Geometry: final body of the model. Coordinates: model frame, mm. Face numbers are marked on the shaded views. A direction names the side the tool comes from. Coordinates: 2 decimals unless noted, no trailing zeros. Order: outer loops, then holes, each group sorted by start corner. A loop starts at its lowest first (then second) coordinate and runs counter-clockwise, first axis right, second up. Notation, with made-up numbers: M -10,-11 L 33,-11 A18 cw 33,2 Z; hole C 61.5,62.25 d1. An arc over 180 degrees is marked long. Use CSV: the item, a comma, the result in double quotes. Start each with the question number.
1. Section query A-A on z = 21.5. State how many separate pieces and enclosed holes the cut face has, and give its area (3 significant figures).
2. Set-up query: the marked faces 4 and 5. Return all of +Z, -Z, +X, -X, +Y, -Y with unobstructed straight access to the full face (end or side cutting, diameter ignored); none if empty.
3. Material intervals for line 1 (Z direction, x = 3.3, y = 9); line 2 (Z direction, x = 1.85, y = -9); line 3 (Z direction, x = 8.5, y = -8.5), sorted ascending.
4. Section query C-C on x = 2. Return the cut outline in (y, z), and give its area (3 significant figures).
5. Pull-direction query (Z, two-part tool) for the marked faces 1, 2 and 3; classes: pulls with the +Z half, pulls with the -Z half, needs draft (parallel to the pull), parting line crosses it, or undercut.
6. First-contact query: P1, Ø15, axis at y = 0.5, z = 10, coming from the +X side; P2, Ø1, axis at x = 8.5, y = 11, coming from the +Z side; P3, Ø8, axis at x = 14, z = 6, coming from the +Y side; P4, Ø1.5, axis at x = 8.5, z = -21, coming from the +Y side. Flat tips, straight axial feed; report the tip coordinate or a pass-through.
7. Section query D-D on y = -0.5. Return the cut outline in (x, z), and give its area (3 significant figures).
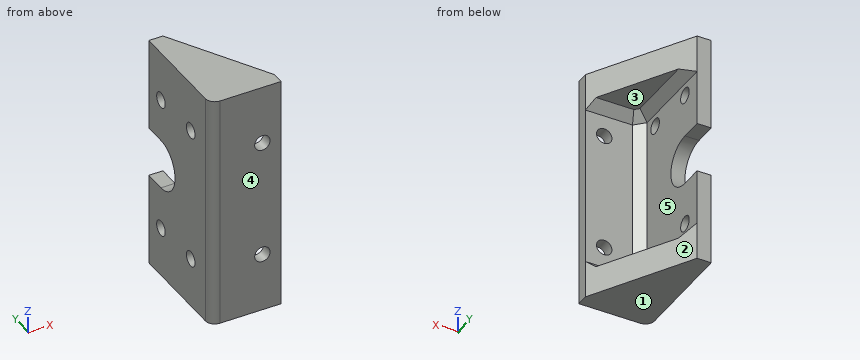
Autodesk Inventor part; units mm, degrees
ref_plane "YZ Plane" through (0, 0, 0) normal (1, 0, 0) x (0, 1, 0)
ref_plane "XZ Plane" through (0, 0, 0) normal (0, 1, 0) x (-1, 0, 0)
ref_plane "XY Plane" through (0, 0, 0) normal (0, 0, 1) x (1, 0, 0)
sketch "Sketch1" plane through (0, 0, 0) normal (1, 0, 0) x (0, 1, 0)
  line L0 (-9, -23) -> (9, -23) construction
  line L1 (9, -23) -> (9, 23) construction
  line L2 (9, 23) -> (-9, 23) construction
  line L3 (-9, 23) -> (-9, -23) construction
  line L4 (-9, -23) -> (9, 23) construction
  line L5 (9, -23) -> (-9, 23) construction
  circle A0 centre (9, 23) radius 2.6
  circle A1 centre (9, -23) radius 2.6
  circle A2 centre (-9, -23) radius 2.6
  circle A3 centre (-9, 23) radius 2.6
  circle A4 centre (9, 23) radius 7.3625 construction
  circle A5 centre (9, -23) radius 7.3625 construction
  circle A6 centre (-9, -23) radius 7.3625 construction
  circle A7 centre (-9, 23) radius 7.3625 construction
  line L6 (16.3625, 30.3625) -> (-21, 30.3625)
  line L7 (-21, 30.3625) -> (-21, -30.3625)
  line L8 (-21, -30.3625) -> (16.3625, -30.3625)
  line L9 (16.3625, -30.3625) -> (16.3625, 30.3625)
  point P0 (0, 0)
  dimension "d0" = 5.2
  dimension "d1" = 46
  dimension "d2" = 18
  dimension "d3" = 4.7625
  dimension "d7" = 12
extrude "Extrusion1" add sketch "Sketch1" along normal blind 4.7625
sketch "Sketch4" plane through (4.7625, 0, 0) normal (1, 0, 0) x (0, 0, -1)
  arc A0 (-8.5, 9) -> (8.5, 9) centre (0, 9) ccw
  circle A1 centre (-23, 9) radius 2.6
  line L0 (8.5, 9) -> (8.5, 16.3625)
  line L1 (30.3625, 16.3625) -> (-30.3625, 16.3625)
  line L2 (-8.5, 9) -> (-8.5, 16.3625)
  point P0 (0, 0)
  point P1 (27.1875, 16.3625)
  point P2 (-27.1875, 16.3625)
  dimension "d21" = 17
extrude "Extrusion5" cut sketch "Sketch4" against normal through all contours L2 L1 L0 A0
sketch "Sketch5" plane through (4.7625, 0, 0) normal (1, 0, 0) x (0, 0, -1)
  line L0 (30.3625, 16.3625) -> (8.5, 16.3625)
  line L1 (-30.3625, 16.3625) -> (-30.3625, -21)
  line L2 (-30.3625, -21) -> (30.3625, -21)
  line L3 (30.3625, -21) -> (30.3625, 16.3625)
  line L4 (-8.5, 16.3625) -> (-30.3625, 16.3625)
  line L5 (8.5, 16.3625) -> (8.5, 9)
  arc A0 (-8.5, 9) -> (8.5, 9) centre (0, 9) ccw
  line L6 (-8.5, 9) -> (-8.5, 16.3625)
  circle A1 centre (-23, -9) radius 2.6
  circle A2 centre (23, -9) radius 2.6
  circle A3 centre (23, 9) radius 2.6
  circle A4 centre (-23, 9) radius 2.6
  line L7 (30.3625, -21) -> (30.3625, 13.1875)
  line L8 (-30.3625, -21) -> (30.3625, -21)
  line L9 (30.3625, -21) -> (30.3625, -17)
  line L10 (30.3625, -17) -> (-30.3625, -17)
  line L11 (-30.3625, -17) -> (-30.3625, -21)
  point P0 (0, 0)
  point P1 (30.3625, -17.825)
  point P2 (30.3625, -17)
  point P3 (-30.3625, -17)
  dimension "d29" = 4
extrude "Extrusion6" add sketch "Sketch5" along normal blind 19.05 contours L3 L2 L1 L10
sketch "Sketch6" plane through (4.7625, -17, 30.3625) normal (0, 1, 0) x (1, 0, 0)
  circle A0 centre (12.7, 10.3625) radius 2.6
  circle A1 centre (12.7, 50.3625) radius 2.6
  line L0 (0, 9.9625) -> (0, 4.7625)
  line L1 (0, 0) -> (0, 60.725)
  line L2 (19.05, 60.725) -> (19.05, 0)
  point P0 (-4.7625, 30.3625)
  point P1 (19.05, 30.3625)
  point P2 (19.05, 30.3625)
  dimension "d32" = 5.2
  dimension "d34" = 20
  dimension "d35" = 20
  dimension "d40" = 6.35
extrude "Extrusion7" cut sketch "Sketch6" against normal through all
sketch "Sketch12" plane through (0, -21, -30.3625) normal (0, 0, -1) x (-1, 0, 0)
  line L0 (0, 0) -> (0, 37.3625)
  line L1 (0, 37.3625) -> (-4.7625, 37.3625)
  line L2 (-4.7625, 4) -> (-4.7625, 37.3625)
  line L3 (-4.7625, 4) -> (-23.8125, 4)
  line L4 (-23.8125, 0) -> (-23.8125, 4)
  line L5 (0, 0) -> (-23.8125, 0)
  line L6 (-23.8125, 0) -> (-23.8125, 4)
  line L7 (-4.7625, 37.3625) -> (-23.8125, 4)
  point P0 (0, 21)
extrude "Extrusion13" add sketch "Sketch12" along normal blind 9.525
sketch "Sketch13" plane through (0, -21, 30.3625) normal (0, 0, 1) x (1, 0, 0)
  line L0 (4.7625, 4) -> (23.8125, 4)
  line L1 (4.7625, 37.3625) -> (23.8125, 4)
  line L2 (4.7625, 4) -> (4.7625, 37.3625)
  line L3 (0, 37.3625) -> (0, 0)
  line L4 (0, 0) -> (23.8125, 0)
  line L5 (23.8125, 4) -> (23.8125, 0)
  line L6 (4.7625, 4) -> (23.8125, 4)
  line L7 (4.7625, 37.3625) -> (4.7625, 4)
  line L8 (0, 37.3625) -> (4.7625, 37.3625)
  point P0 (0, 21)
  point P1 (23.8125, 4)
  point P2 (4.7625, 37.3625)
extrude "Extrusion14" add sketch "Sketch13" along normal blind 9.525
chamfer "Chamfer1" distance 3.175 angle 45 1 edges at (4.7625, -17, 0)
chamfer "Chamfer2" distance 3.175 angle 45 6 edges at (15.875, -17, 30.3625) (6.35, -15.4125, 30.3625) (4.7625, 1.2687, 30.3625) (4.7625, 1.2688, -30.3625) (6.35, -15.4125, -30.3625) (15.875, -17, -30.3625)
fillet "Fillet9" radius 3.175 1 edges at (0, -21, 0)
properties part number "CNC-022-XAxisBallScrewStabilizerMount" material "ABS Plastic"
Results list:
1,separate pieces,"4"
1,enclosed holes,"0"
1,area,"200 mm²"
2,face 4,"+Z, -Z, +X, -X, -Y"
2,face 5,"+X, +Y"
3,line 1,"z = -39.89 to -25.6, -20.4 to -8.5, 8.5 to 20.4, 25.6 to 39.89"
3,line 2,"z = -39.89 to -25.6, -20.4 to 20.4, 25.6 to 39.89"
3,line 3,"z = -39.89 to -30.36, 30.36 to 39.89"
4,outline,"M -20.77,-39.89 L 16.36,-39.89 L 16.36,-8.5 L 9,-8.5 A8.5 cw 9,8.5 L 16.36,8.5 L 16.36,39.89 L -20.77,39.89 Z; hole C -9,-23 d5.2; hole C -9,23 d5.2; hole C 9,-23 d5.2; hole C 9,23 d5.2"
4,area,"2,640 mm²"
5,face 1,"pulls with the -Z half"
5,face 2,"needs draft"
5,face 3,"undercut"
6,P1,"stops at x = 4.76"
6,P2,"passes through"
6,P3,"stops at y = -17"
6,P4,"stops at y = -16.81"
7,outline,"M 0,-39.89 L 14.39,-39.89 L 14.39,-30.36 L 7.94,-30.36 L 4.76,-27.19 L 4.76,27.19 L 7.94,30.36 L 14.39,30.36 L 14.39,39.89 L 0,39.89 Z"
7,area,"573 mm²"
